Can you work these out from the drawing? Everything is in mm from the part's minimum corner. Give positions to 0.01 mm unless a question says otherwise; leave off trailing zeros. Order: outer loops, then holes, each group sorted by start corner. A loop starts at its lowest first (then second) coordinate and runs counter-clockwise, first axis right, second up. Notation, with made-up numbers: (-21, 19.25) -> (34, 19.25) arc R9 ccw to (34, 24.25) -> close; hole circle Ø9 at (-25, 1.5). An arc over 180 degrees is marked (long way). Answer as CSV lines item,"result". Start each with the question number.
(1) I need wall thicknesses on L1, parallel to Y at x = 7, z = 1.9; L2, parallel to X at y = 3.25, z = 1.75; L3, parallel to Z at x = 24, y = 3.75. Which ranges of each line are inside material? Lowest first, please.
(2) I want a section at D-D (x = 7.5). Please give me the cut outline in (y, z), plus the area to 3 significant figures.
(3) I want a section at C-C (z = 0.6). Please give me the cut outline in (x, y), plus the area to 3 significant figures.
(4) I want a section at B-B (x = 44). Please give me the cut outline in (y, z), plus the area to 3 significant figures.
(5) I want a section at A-A (y = 4). Give the number of separate pieces and of enclosed holes in the cut face, plus the area to 3 significant figures.
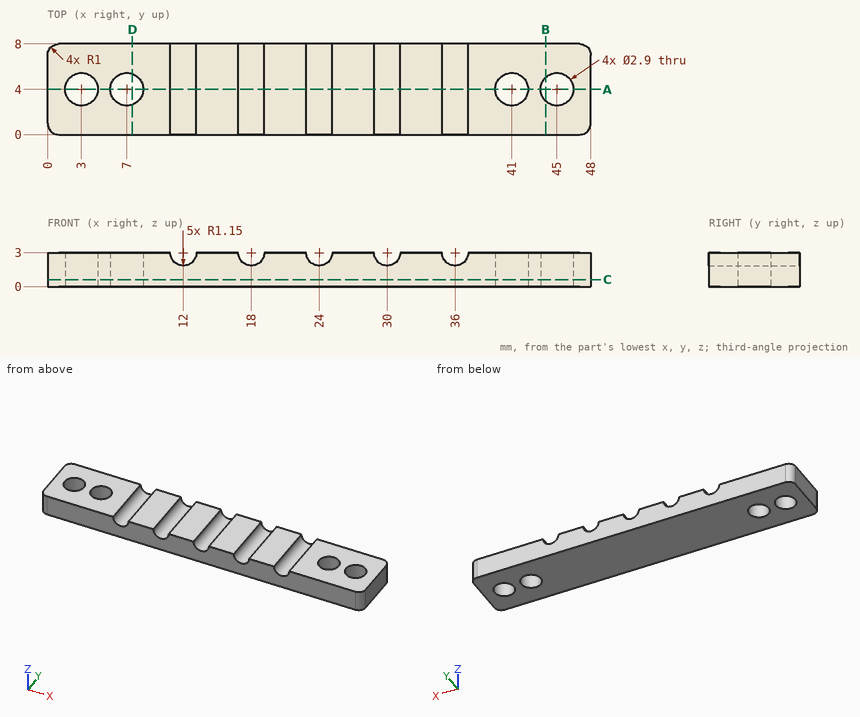
Final values:
1,L1,"0 to 2.55, 5.45 to 8"
1,L2,"0 to 1.76, 4.24 to 5.76, 8.24 to 39.76, 42.24 to 43.76, 46.24 to 48"
1,L3,"0 to 1.85"
2,outline,"(0, 0) -> (2.64, 0) -> (2.64, 3) -> (0, 3) -> close; (5.36, 0) -> (8, 0) -> (8, 3) -> (5.36, 3) -> close"
2,area,"15.8 mm²"
3,outline,"(0, 1) arc R1 ccw to (1, 0) -> (47, 0) arc R1 ccw to (48, 1) -> (48, 7) arc R1 ccw to (47, 8) -> (1, 8) arc R1 ccw to (0, 7) -> close; hole circle Ø2.9 at (3, 4); hole circle Ø2.9 at (7, 4); hole circle Ø2.9 at (41, 4); hole circle Ø2.9 at (45, 4)"
3,area,"357 mm²"
4,outline,"(0, 0) -> (2.95, 0) -> (2.95, 3) -> (0, 3) -> close; (5.05, 0) -> (8, 0) -> (8, 3) -> (5.05, 3) -> close"
4,area,"17.7 mm²"
5,separate pieces,"5"
5,enclosed holes,"0"
5,area,"98.8 mm²"
